The model under review builds one solid part; all positions refer to its coordinate system, in mm. Give positions to 0.01 mm unless a question says otherwise; leave off trailing zeros. Order: outer loops, then holes, each group sorted by start corner. A loop starts at its lowest first (then second) coordinate and runs counter-clockwise, first axis right, second up.
```python
from build123d import *

# Parameters (mm, degrees)
F0_W        = 50
F0_H        = 50
F0_W_2      = 44
F0_H_2      = 44
F1_DEPTH    = 1430
F2_T1_DEPTH = 307.1682987966


# Not quite as in the source:
# - a fillet or chamfer that OpenCascade refuses, or shapes differently, is made with other operations: its cross-section is extruded or revolved along the edge and cut away or added


with BuildPart() as f1:
    # F0 (on Top) → F1 (new body)
    with BuildSketch(Plane.XY):
        with Locations((25, 25)):
            Rectangle(F0_W, F0_H)
        with Locations((25, 25)):
            Rectangle(F0_W_2, F0_H_2, mode=Mode.SUBTRACT)
    extrude(amount=F1_DEPTH)

    # F2: chamfer of 50 on 2 edges, made by hand

    # F2_s2 → F2_t1 (cut)
    with BuildSketch(Plane.XZ.offset(-178.5841493983)):
        Polygon((0, 50), (50, 0), (0, 0), align=None)
        Polygon((0, 1380), (50, 1430), (0, 1430), align=None)
    extrude(amount=F2_T1_DEPTH, mode=Mode.SUBTRACT)


solid = f1.part
```
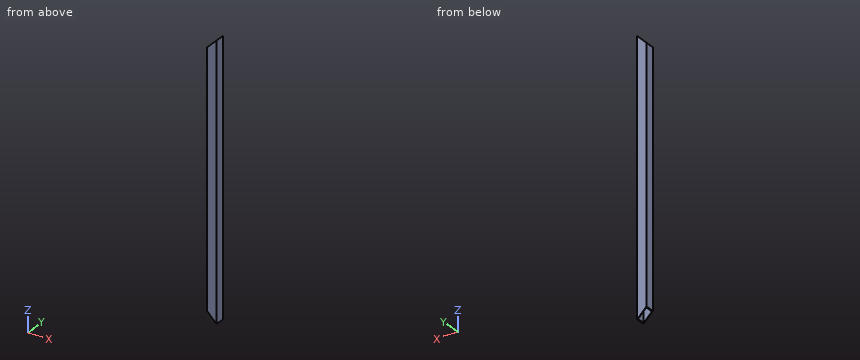
Item 1: Take a section at A-A (x = 19). Give the boundary of the cut face in (y, z), and give its area (3 significant figures).
Values found:
outline: (0, 31) - (3, 31) - (3, 1399) - (0, 1399) - close; (47, 31) - (50, 31) - (50, 1399) - (47, 1399) - close
area: 8,210 mm2
Item 2: Take a section at B-B (z = 584). Give the boundary of the cut face in (x, y).
Values found:
outline: (0, 0) - (50, 0) - (50, 50) - (0, 50) - close; hole (3, 3) - (47, 3) - (47, 47) - (3, 47) - close
Item 3: Clearance check with a flat-ended pin moving along its axis: pin 1 Ø6 at (x, y) = (5.5, 35) entering from -Z. State where the tip first meets the part, or that it passes through.
Values found:
pin 1: stops at z = 47
Item 4: For line 1 (X direction, y = 23, z = 539), list the stretches that pass through material, from the lowest coordinate up.
Values found:
line 1: x = 0 to 3, 47 to 50
Item 5: Take a section at C-C (y = 37.5). Give the boundary of the cut face in (x, z), and give its area (3 significant figures).
Values found:
outline: (0, 50) - (3, 47) - (3, 1383) - (0, 1380) - close; (47, 3) - (50, 0) - (50, 1430) - (47, 1427) - close
area: 8,280 mm2
